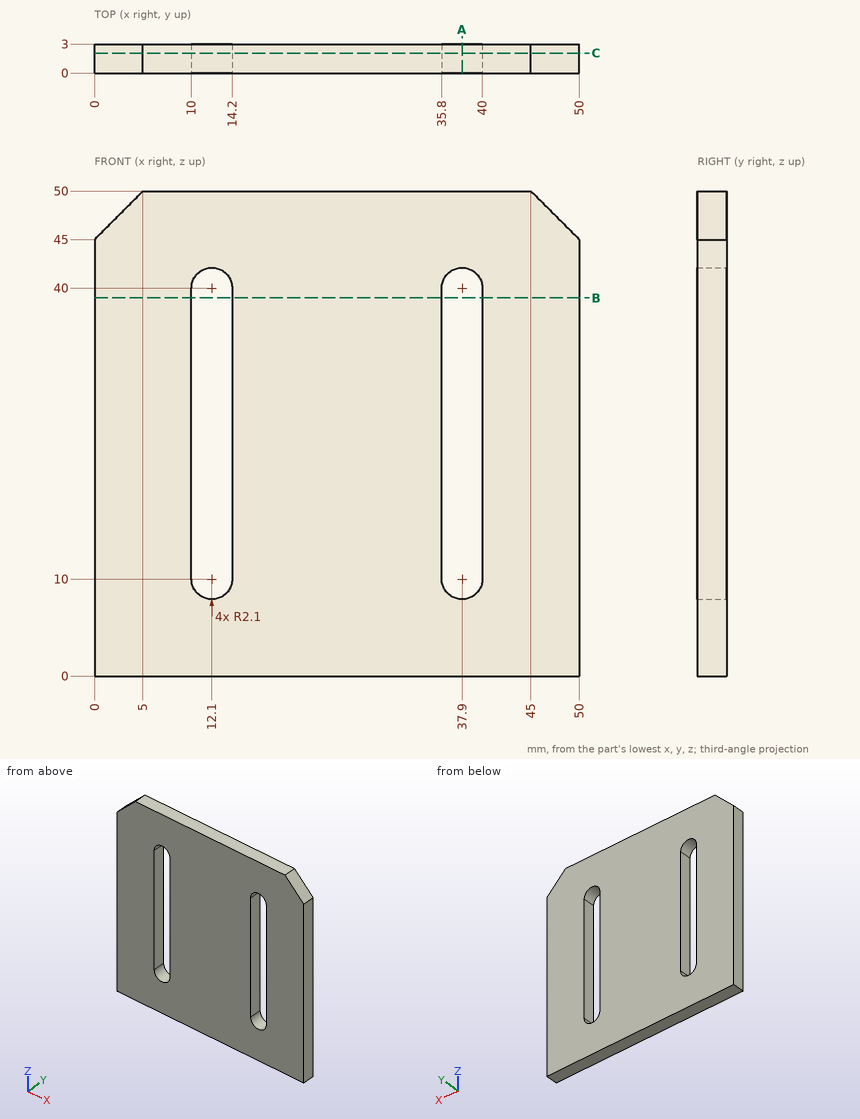
Print and shaded views of the part. All mm, measured from the part's lowest x, y and z. Give positions to 0.01 mm unless a question says otherwise; leave off trailing zeros. Order: outer loops, then holes, each group sorted by start corner. A loop starts at its lowest first (then second) coordinate and runs counter-clockwise, first axis right, second up. Notation, with made-up numbers: (77, -18.5) -> (115, -18.5) arc R32 cw to (115, 11.5) -> close; hole circle Ø7 at (-19.75, 86). An arc over 180 degrees is marked (long way). Use CSV: the item, a comma, the result in double quotes.
1. Band-saw the part on C-C, the plane y = 2.05. Give the cut face in (x, z).
Outcome:
outline,"(0, 0) -> (50, 0) -> (50, 45) -> (45, 50) -> (5, 50) -> (0, 45) -> close; hole (10, 10) arc R2.1 ccw to (14.2, 10) -> (14.2, 40) arc R2.1 ccw to (10, 40) -> close; hole (35.8, 10) arc R2.1 ccw to (40, 10) -> (40, 40) arc R2.1 ccw to (35.8, 40) -> close"
2. Band-saw the part on A-A, the plane x = 37.9. Give the cut face in (y, z), then the cut area to 3 significant figures.
Outcome:
outline,"(0, 0) -> (3, 0) -> (3, 7.9) -> (0, 7.9) -> close; (0, 42.1) -> (3, 42.1) -> (3, 50) -> (0, 50) -> close"
area,"47.4 mm²"
3. Band-saw the part on B-B, the plane z = 39. Give the cut face in (x, y).
Outcome:
outline,"(0, 0) -> (10, 0) -> (10, 3) -> (0, 3) -> close; (14.2, 0) -> (35.8, 0) -> (35.8, 3) -> (14.2, 3) -> close; (40, 0) -> (50, 0) -> (50, 3) -> (40, 3) -> close"
4. Drill centre lines: line 1 along X through (y, z) = (0.5, 38); line 2 along Z through (x, y) = (12, 0.6); line 3 along Z through (x, y) = (3.5, 1.35). Where is each one in solid material? Low to high. Write a range as from..to.
Outcome:
line 1,"0..10, 14.2..35.8, 40..50"
line 2,"0..7.9, 42.1..50"
line 3,"0..48.5"
